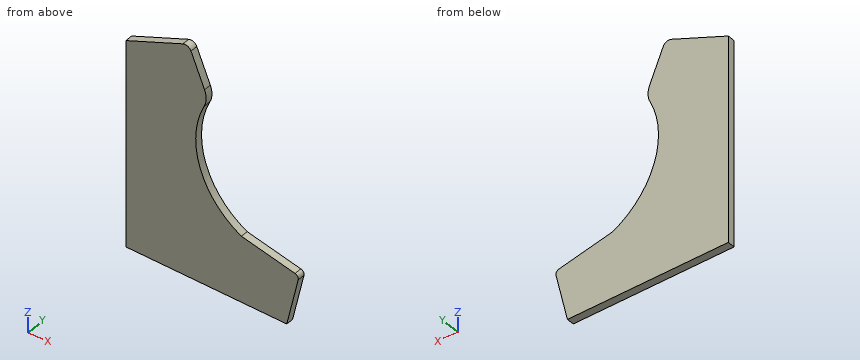
```python
from build123d import *

# Parameters (mm, degrees)
F1_DEPTH = 18


with BuildPart() as f1:
    # F0 (on Front) → F1 (new body)
    with BuildSketch(Plane.XZ):
        with BuildLine():
            Line((0, 500), (0, 0))
            Line((0, 0), (390, 0))
            Line((390, 0), (417.715809, 120.10184))
            ThreePointArc((417.715809, 120.10184), (416.41, 127.716852), (410.067188, 132.12846))
            Line((410.067188, 132.12846), (280, 160))
            ThreePointArc((280, 160), (179.794974, 277.193689), (189.612331, 431.073602))
            ThreePointArc((189.612331, 431.073602), (194.55811, 451.520543), (190.655976, 472.192056))
            Line((190.655976, 472.192056), (157.820855, 550.175469))
            ThreePointArc((157.820855, 550.175469), (149.655778, 558.246), (138.175469, 558.179145))
            Line((138.175469, 558.179145), (0, 500))
        make_face()
    extrude(amount=F1_DEPTH)


solid = f1.part
```
CAD build for the part. Positions are in the model's coordinates, mm. Coordinates: 2 decimals unless noted, no trailing zeros. Write each loop counter-clockwise with the first axis right and the second up, starting at its lowest first coordinate (ties: lowest second). Pieces come first, ordered by that corner, then holes.
(1) Cut at C-C, the plane x = 347. List the corners of the cut face in (y, z).
(2) Cut at B-B, the plane z = 385. List the corners of the cut face in (x, y), and give its area (3 significant figures).
(3) Drill centre lines: probe 1 along X at (y, z) = (-11.5, 455); probe 2 along X at (y, z) = (-15.5, 298); probe 3 along Z at (x, y) = (161, -13) (3 decimals). Where is each one in solid material? Low to high.
(4) Cut at A-A, the plane y = -6.75. List the corners of the cut face in (x, z), and give its area (3 significant figures).
(5) Flat gauge pins, fed straight in: pin 1 (4 mm diameter, centred on x = 341, y = -8.5, fed in from +Z); pin 2 (4 mm diameter, centred on x = 89.5, y = -8.5, fed in from +Z); pin 3 (1 mm diameter, centred on y = -5.5, z = 206, fed in from +X). Where does each tip first touch, or does it go through?
Geometry says:
1. outline: (-18, 0) - (0, 0) - (0, 145.64) - (-18, 145.64) - close
2. outline: (0, -18) - (173.82, -18) - (173.82, 0) - (0, 0) - close
2. area: 3,130 mm2
3. probe 1: x = 0 to 194.53
3. probe 2: x = 0 to 174.05
3. probe 3: z = 0 to 542.625
4. outline: (0, 0) - (390, 0) - (417.72, 120.1) arc R10 ccw to (410.07, 132.13) - (280, 160) arc R205 cw to (189.61, 431.07) arc R50 ccw to (190.66, 472.19) - (157.82, 550.18) arc R15 ccw to (138.18, 558.18) - (0, 500) - close
4. area: 134,000 mm2
5. pin 1: stops at z = 147.36
5. pin 2: stops at z = 538.53
5. pin 3: stops at x = 221.36
